Could you check a few things on this model? Use its own coordinates, in mm. Face numbers are marked on the shaded views. A direction names the side the tool comes from. Give positions to 0.01 mm unless a question says otherwise; leave off trailing zeros. Write each loop counter-clockwise with the first axis right and the second up, starting at its lowest first coordinate (ties: lowest second). Pieces come first, ordered by that corner, then holes. Notation, with made-up numbers: (-8.5, 85) - (46.5, 85) arc R23 cw to (46.5, 101) - close; hole circle Ø7 at (46.5, 33). An arc over 180 degrees is marked (long way). Answer as CSV lines item,"result". Start each with the question number.
Q1. Imagine slicing it at B-B on x = 15.5. List the corners of the cut face in (y, z) for me.
Q2. We'd pull the mould along X, two halves only. Please class the marked faces 1, 2, 3 and 4: pulls with the +X half, pulls with the -X half, needs draft (parallel to the pull), parting line crosses it, or undercut.
Q3. Imagine slicing it at A-A on z = 27.5. List the corners of the cut face in (x, y) for me, and give its area (3 significant figures).
Q4. Imagine slicing it at D-D on y = -3.5. List the corners of the cut face in (x, z) for me.
Q5. On a 3-axis mill with a long thin cutter (end or side, diameter ignored), from which of +Z, -Z, +X, -X, +Y, -Y can I reach the whole of each face in a straight line? I mean the marked faces 5, 6 and 7. Say none if no direction works.
Q6. If I drill on line 1 along X through (y, z) = (-26, 15); line 2 along X through (y, z) = (-4.5, 2.5); line 3 along Y through (x, z) = (44, 3.5), over which ranges is the centre line in solid material (lowest first)?
Q7. Will these pins go through, and if not, where does the flat tip stop? pin 1 Ø4 at (x, z) = (5.5, 21) entering from -Y; pin 2 Ø8.5 at (x, z) = (3.5, 24.5) entering from +Y.
Q8. Imagine slicing it at C-C on y = -21.5. List the corners of the cut face in (x, z) for me.
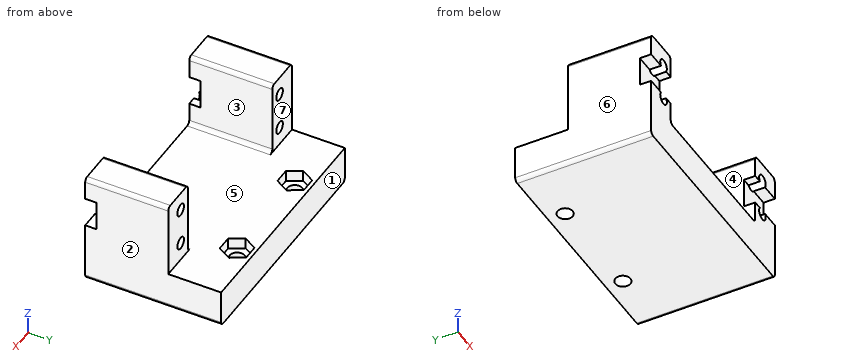
```python
from build123d import *

# Parameters (mm, degrees)
SKETCH1_W           = 60
SKETCH1_H           = 36
SKETCH1_R           = 2
BOSS_EXTRUDE1_DEPTH = 10
SKETCH2_W           = 9.5
SKETCH2_H           = 20
BOSS_EXTRUDE2_DEPTH = 22
CUT_EXTRUDE1_REACH  = 72.597
SKETCH3_R           = 1.6
CUT_EXTRUDE2_DEPTH  = 3
LPATTERN1_COUNT     = 2
LPATTERN1_PITCH     = 28
FILLET1_R           = 1
SKETCH6_W           = 8
SKETCH6_H           = 3
CUT_EXTRUDE3_DEPTH  = 77.131465243


with BuildPart() as part:
    # Sketch1 → Boss-Extrude1 (new body)
    with BuildSketch(Plane.XY):
        with Locations((30, -18)):
            Rectangle(SKETCH1_W, SKETCH1_H)
        with Locations((16, -4.5)):
            Circle(SKETCH1_R, mode=Mode.SUBTRACT)
        with Locations((44, -4.5)):
            Circle(SKETCH1_R, mode=Mode.SUBTRACT)
    extrude(amount=BOSS_EXTRUDE1_DEPTH)

    # Sketch2 → Boss-Extrude2 (add)
    with BuildSketch(Plane.XZ.offset(36)):
        with Locations((4.75, 20)):
            Rectangle(SKETCH2_W, SKETCH2_H)
        with Locations((55.25, 20)):
            Rectangle(SKETCH2_W, SKETCH2_H)
    extrude(amount=-BOSS_EXTRUDE2_DEPTH)

    # Sketch3 → Cut-Extrude1 (cut, up to next)
    with BuildSketch(Plane(origin=(0, -14, 0), x_dir=(1, 0, 0), z_dir=(0, 1, 0)), mode=Mode.PRIVATE) as cut_extrude1_sk1:
        with Locations(Location((6, -15, 0), (0, 0, 270))):
            Circle(SKETCH3_R)
    cut_extrude1_tool1 = extrude(cut_extrude1_sk1.sketch, amount=-CUT_EXTRUDE1_REACH, mode=Mode.PRIVATE) & part.part
    # Sketch3 → Cut-Extrude1 (cut, up to next)
    with BuildSketch(Plane(origin=(0, -14, 0), x_dir=(1, 0, 0), z_dir=(0, 1, 0)), mode=Mode.PRIVATE) as cut_extrude1_sk2:
        with Locations(Location((54, -15, 0), (0, 0, 270))):
            Circle(SKETCH3_R)
    cut_extrude1_tool2 = extrude(cut_extrude1_sk2.sketch, amount=-CUT_EXTRUDE1_REACH, mode=Mode.PRIVATE) & part.part
    # Sketch3 → Cut-Extrude1 (cut, up to next)
    with BuildSketch(Plane(origin=(0, -14, 0), x_dir=(1, 0, 0), z_dir=(0, 1, 0)), mode=Mode.PRIVATE) as cut_extrude1_sk3:
        with Locations(Location((54, -25, 0), (0, 0, 270))):
            Circle(SKETCH3_R)
    cut_extrude1_tool3 = extrude(cut_extrude1_sk3.sketch, amount=-CUT_EXTRUDE1_REACH, mode=Mode.PRIVATE) & part.part
    # Sketch3 → Cut-Extrude1 (cut, up to next)
    with BuildSketch(Plane(origin=(0, -14, 0), x_dir=(1, 0, 0), z_dir=(0, 1, 0)), mode=Mode.PRIVATE) as cut_extrude1_sk4:
        with Locations(Location((6, -25, 0), (0, 0, 270))):
            Circle(SKETCH3_R)
    cut_extrude1_tool4 = extrude(cut_extrude1_sk4.sketch, amount=-CUT_EXTRUDE1_REACH, mode=Mode.PRIVATE) & part.part
    add(cut_extrude1_tool1.solids().sort_by_distance((6, -14, 15))[0], mode=Mode.SUBTRACT)
    add(cut_extrude1_tool2.solids().sort_by_distance((54, -14, 15))[0], mode=Mode.SUBTRACT)
    add(cut_extrude1_tool3.solids().sort_by_distance((54, -14, 25))[0], mode=Mode.SUBTRACT)
    add(cut_extrude1_tool4.solids().sort_by_distance((6, -14, 25))[0], mode=Mode.SUBTRACT)

    # Sketch4 → Cut-Extrude2 (cut)
    with BuildSketch(Plane.XY.offset(10)):
        Polygon((13.979274058, -1), (11.958548116, -4.5), (13.979274058, -8), (18.020725942, -8), (20.041451884, -4.5), (18.020725942, -1), align=None)
    cut_extrude2 = extrude(amount=-CUT_EXTRUDE2_DEPTH, mode=Mode.SUBTRACT)

    # LPattern1: Cut-Extrude2 ×2
    with Locations(*[(i * LPATTERN1_PITCH, 0, 0) for i in range(1, LPATTERN1_COUNT)]):
        add(cut_extrude2, mode=Mode.SUBTRACT)

    # Fillet1
    fillet1_edges = [part.edges().sort_by_distance(p)[0] for p in [
        (0, -25, 30),
        (9.5, -25, 30),
        (9.5, -25, 10),
        (60, -25, 30),
        (50.5, -25, 10),
        (50.5, -25, 30),
        (60, -18, 0),
        (0, -18, 0),
    ]]
    fillet(fillet1_edges, radius=FILLET1_R)

    # Sketch6 → Cut-Extrude3 (cut, through all)
    with BuildSketch(Plane(origin=(60, 0, 0), x_dir=(0, 0, -1), z_dir=(1, 0, 0))):
        with Locations((-20, -34.5)):
            Rectangle(SKETCH6_W, SKETCH6_H)
    extrude(amount=-CUT_EXTRUDE3_DEPTH, mode=Mode.SUBTRACT)


solid = part.part
```
Conclusion:
1,outline,"(-36, 0) - (-6.44, 0) - (-6.44, 7) - (-8, 7) - (-8, 10) - (-36, 10) - close; (-2.56, 0) - (0, 0) - (0, 10) - (-1, 10) - (-1, 7) - (-2.56, 7) - close"
2,face 1,"needs draft"
2,face 2,"pulls with the +X half"
2,face 3,"undercut"
2,face 4,"undercut"
3,outline,"(0, -36) - (9.5, -36) - (9.5, -14) - (0, -14) - close; (50.5, -36) - (60, -36) - (60, -14) - (50.5, -14) - close"
3,area,"418 mm^2"
4,outline,"(0, 1) arc R1 ccw to (1, 0) - (14.27, 0) - (14.27, 7) - (12.54, 7) - (12.54, 10) - (0, 10) - close; (17.73, 0) - (42.27, 0) - (42.27, 7) - (40.54, 7) - (40.54, 10) - (19.46, 10) - (19.46, 7) - (17.73, 7) - close; (45.73, 0) - (59, 0) arc R1 ccw to (60, 1) - (60, 10) - (47.46, 10) - (47.46, 7) - (45.73, 7) - close"
5,face 5,"+Z, +Y"
5,face 6,"+Z, -Z, -X, +Y, -Y"
5,face 7,"+Z, +X, -X, +Y"
6,line 1,"0 to 4.4, 7.6 to 9.5, 50.5 to 52.4, 55.6 to 60"
6,line 2,"0 to 14, 18 to 42, 46 to 60"
6,line 3,"-36 to -6.5, -2.5 to 0"
7,pin 1,"y = -33"
7,pin 2,"y = -14"
8,outline,"(0, 1) arc R1 ccw to (1, 0) - (59, 0) arc R1 ccw to (60, 1) - (60, 29) arc R1 ccw to (59, 30) - (51.5, 30) arc R1 ccw to (50.5, 29) - (50.5, 11) arc R1 cw to (49.5, 10) - (10.5, 10) arc R1 cw to (9.5, 11) - (9.5, 29) arc R1 ccw to (8.5, 30) - (1, 30) arc R1 ccw to (0, 29) - close; hole circle Ø3.2 at (6, 15); hole circle Ø3.2 at (6, 25); hole circle Ø3.2 at (54, 15); hole circle Ø3.2 at (54, 25)"
